Here's how the part is built. I have some questions about the finished solid (model axes, mm). Give positions to 0.01 mm unless a question says otherwise; leave off trailing zeros. Order: outer loops, then holes, each group sorted by start corner. A loop starts at its lowest first (then second) coordinate and runs counter-clockwise, first axis right, second up. Notation, with made-up numbers: (18, 70) - (56, 70) arc R12 cw to (56, 93) - close; hole circle Ø9 at (32, 73.5). An arc over 180 degrees is marked (long way). One line per question, with ' | ' between items.
from build123d import *

# Parameters (mm, degrees)
AUFSATZ_LINEAR_AUSTRAGEN1_DEPTH = 4
SCHNITT_LINEAR_AUSTRAGEN1_REACH = 6
SKIZZE2_R                       = 8
SKIZZE2_R_2                     = 2.141321697
SCHNITT_LINEAR_START            = -4
SCHNITT_LINEAR_AUSTRAGEN2_DEPTH = 4
AUFSATZ_LINEAR_AUSTRAGEN3_DEPTH = 4
AUFSATZ_LINEAR_AUSTRAGEN4_DEPTH = 4
SCHNITT_LINEAR_AUSTRAGEN3_REACH = 6
SKIZZE6_R                       = 1.55


with BuildPart() as part:
    # Skizze1 → Aufsatz-Linear austragen1 (new body)
    with BuildSketch(Plane.XY):
        with BuildLine():
            Line((28.570550732, -10.430515814), (-71.429449268, -10.430515814))
            ThreePointArc((-71.429449268, -10.430515814), (-93.5, 0), (-71.429449268, 10.430515814))
            Line((-71.429449268, 10.430515814), (-65.575289804, 10.430515814))
            ThreePointArc((-65.575289804, 10.430515814), (-61.49939442, 6.35462043), (-57.423499036, 10.430515814))
            Line((-57.423499036, 10.430515814), (28.570550732, 10.430515814))
            ThreePointArc((28.570550732, 10.430515814), (39.001066546, 0), (28.570550732, -10.430515814))
        make_face()
    extrude(amount=AUFSATZ_LINEAR_AUSTRAGEN1_DEPTH)

    # Skizze2 → Schnitt-Linear austragen1 (cut, up to next)
    with BuildSketch(Plane.XY.offset(4), mode=Mode.PRIVATE) as schnitt_linear_austragen1_sk1:
        with Locations((-80, 0)):
            Circle(SKIZZE2_R)
    schnitt_linear_austragen1_tool1 = extrude(schnitt_linear_austragen1_sk1.sketch, amount=-SCHNITT_LINEAR_AUSTRAGEN1_REACH, mode=Mode.PRIVATE) & part.part
    add(schnitt_linear_austragen1_tool1.solids().sort_by_distance((-80, 0, 4))[0], mode=Mode.SUBTRACT)
    # Skizze2 → Schnitt-Linear austragen1 (cut, up to next)
    with BuildSketch(Plane.XY.offset(4), mode=Mode.PRIVATE) as schnitt_linear_austragen1_sk2:
        with Locations((-56.152824314, 1.105869461)):
            Circle(SKIZZE2_R_2)
    schnitt_linear_austragen1_tool2 = extrude(schnitt_linear_austragen1_sk2.sketch, amount=-SCHNITT_LINEAR_AUSTRAGEN1_REACH, mode=Mode.PRIVATE) & part.part
    add(schnitt_linear_austragen1_tool2.solids().sort_by_distance((-56.152824, 1.105869, 4))[0], mode=Mode.SUBTRACT)
    # Skizze2 → Schnitt-Linear austragen1 (cut, up to next)
    with BuildSketch(Plane.XY.offset(4), mode=Mode.PRIVATE) as schnitt_linear_austragen1_sk3:
        Polygon((14.803847577, 4.033585801), (20, 7.033585801), (22, 3.569484186), (16.803847577, 0.569484186), align=None)
    schnitt_linear_austragen1_tool3 = extrude(schnitt_linear_austragen1_sk3.sketch, amount=-SCHNITT_LINEAR_AUSTRAGEN1_REACH, mode=Mode.PRIVATE) & part.part
    add(schnitt_linear_austragen1_tool3.solids().sort_by_distance((18.401924, 3.801535, 4))[0], mode=Mode.SUBTRACT)

    # Skizze3 → Schnitt-Linear austragen2 (cut)
    with BuildSketch(Plane.XY.offset(4).offset(SCHNITT_LINEAR_START)):
        Polygon((34.526391185, 28.400642866), (53.593329276, -4.624262653), (24.786074739, -21.256138815), (17.669872981, -8.930515814), (28.92820323, -2.430515814), (18.92820323, 14.889992262), (7.669872981, 8.389992262), (5.719136647, 11.768766704), align=None)
    extrude(amount=SCHNITT_LINEAR_AUSTRAGEN2_DEPTH, mode=Mode.SUBTRACT)

    # Skizze4 → Aufsatz-Linear austragen3 (add)
    with BuildSketch(Plane.XY):
        with BuildLine():
            Line((11.204163448, 10.430515814), (18.92820323, 14.889992262))
            ThreePointArc((18.92820323, 14.889992262), (20.44584132, 15.089793107), (21.660254038, 14.157941454))
            Line((21.660254038, 14.157941454), (29.660254038, 0.301534994))
            ThreePointArc((29.660254038, 0.301534994), (29.860054883, -1.216103097), (28.92820323, -2.430515814))
            Line((28.92820323, -2.430515814), (21.502883158, 10.430515814))
            Line((21.502883158, 10.430515814), (11.204163448, 10.430515814))
        make_face()
    extrude(amount=AUFSATZ_LINEAR_AUSTRAGEN3_DEPTH)

    # Skizze5 → Aufsatz-Linear austragen4 (add)
    with BuildSketch(Plane.XY.offset(4)):
        with BuildLine():
            Line((-63.815140393, -10.430515814), (-53.843758142, -10.430515814))
            ThreePointArc((-53.843758142, -10.430515814), (-58.829449268, -15.808515814), (-63.815140393, -10.430515814))
        make_face()
    extrude(amount=-AUFSATZ_LINEAR_AUSTRAGEN4_DEPTH)

    # Skizze6 → Schnitt-Linear austragen3 (cut, up to next)
    with BuildSketch(Plane.XY.offset(4), mode=Mode.PRIVATE) as schnitt_linear_austragen3_sk1:
        with Locations((-58.663449268, -12.012515814)):
            Circle(SKIZZE6_R)
    schnitt_linear_austragen3_tool1 = extrude(schnitt_linear_austragen3_sk1.sketch, amount=-SCHNITT_LINEAR_AUSTRAGEN3_REACH, mode=Mode.PRIVATE) & part.part
    add(schnitt_linear_austragen3_tool1.solids().sort_by_distance((-58.663449, -12.012516, 4))[0], mode=Mode.SUBTRACT)
    # Skizze6 → Schnitt-Linear austragen3 (cut, up to next)
    with BuildSketch(Plane.XY.offset(4), mode=Mode.PRIVATE) as schnitt_linear_austragen3_sk2:
        with Locations((-43.404449268, -3.025515814)):
            Circle(SKIZZE6_R)
    schnitt_linear_austragen3_tool2 = extrude(schnitt_linear_austragen3_sk2.sketch, amount=-SCHNITT_LINEAR_AUSTRAGEN3_REACH, mode=Mode.PRIVATE) & part.part
    add(schnitt_linear_austragen3_tool2.solids().sort_by_distance((-43.404449, -3.025516, 4))[0], mode=Mode.SUBTRACT)


solid = part.part
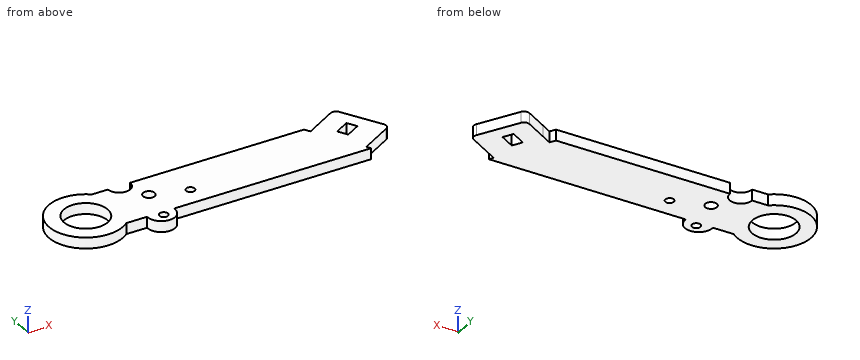
1) I'm going to push flat-ended pins straight in: P1, Ø2, axis at x = -20.5, y = 4.5, coming from the -Z side; P2, Ø2, axis at y = -2, z = 1.5, coming from the +X side; P3, Ø1.2, axis at x = -7.5, z = 2, coming from the -Y side. Where does each tip first touch, or does it pass through?
Model answer:
P1: stops at z = 0 | P2: stops at x = 29.91 | P3: stops at y = -10.43
2) I want a section at C-C (x = -37). List the corners of the cut face in (y, z) for me.
Model answer:
outline: (-10.43, 0) - (10.43, 0) - (10.43, 4) - (-10.43, 4) - close
3) Please list where these lines run through material, in increasing order: L1, parallel to X at y = 1.5, z = 2.75; L2, parallel to X at y = 3.5, z = 1.1; L3, parallel to X at y = -11, z = 3.65.
Model answer:
L1: x = -93.42 to -87.86, -72.14 to -58.26, -54.05 to 16.27, 18.42 to 28.97 | L2: x = -93.04 to -87.19, -72.81 to 15.11, 21.88 to 27.81 | L3: x = -87.83 to -72.17, -63.83 to -59.84, -57.49 to -53.83
4) I want a section at A-A (x = -80). List the corners of the cut face in (y, z) for me, plus the area to 3 significant figures.
Model answer:
outline: (-13.5, 0) - (-8, 0) - (-8, 4) - (-13.5, 4) - close; (8, 0) - (13.5, 0) - (13.5, 4) - (8, 4) - close | area: 44.0 mm2
5) I want a section at B-B (z = 1.35). List the corners of the cut face in (x, y) for me.
Model answer:
outline: (-71.43, -10.43) - (-63.82, -10.43) arc R5 ccw (long way) to (-53.84, -10.43) - (18.54, -10.43) - (17.67, -8.93) - (28.93, -2.43) arc R2 ccw to (29.66, 0.3) - (21.66, 14.16) arc R2 ccw to (18.93, 14.89) - (7.67, 8.39) - (6.49, 10.43) - (-57.42, 10.43) arc R4.08 cw to (-65.58, 10.43) - (-71.43, 10.43) arc R13.5 ccw (long way) to start; hole circle Ø16 at (-80, 0); hole circle Ø3.1 at (-58.66, -12.01); hole circle Ø4.28 at (-56.15, 1.11); hole circle Ø3.1 at (-43.4, -3.03); hole (14.8, 4.03) - (16.8, 0.57) - (22, 3.57) - (20, 7.03) - close
